Model file for the job. Use its own axes, mm. Face numbers are marked on the shaded views. A direction names the side the tool comes from. Round coordinates to 2 decimals unless told otherwise and drop trailing zeros. Write each loop counter-clockwise with the first axis right and the second up, starting at its lowest first coordinate (ties: lowest second). Pieces come first, ordered by that corner, then holes.
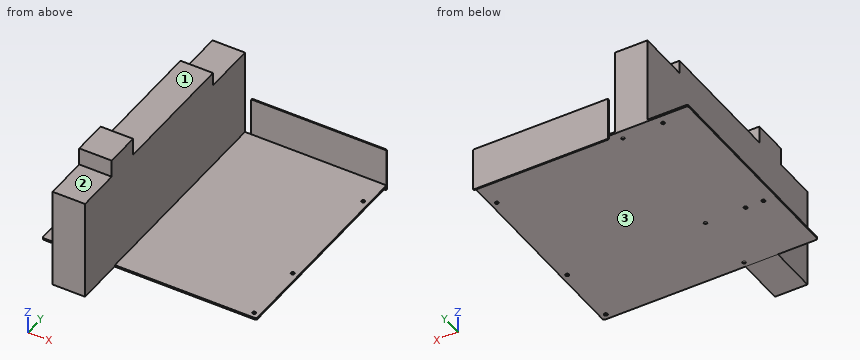
Autodesk Inventor part; units mm, degrees
ref_plane "YZ Plane" through (0, 0, 0) normal (1, 0, 0) x (0, 1, 0)
ref_plane "XZ Plane" through (0, 0, 0) normal (0, 1, 0) x (-1, 0, 0)
ref_plane "XY Plane" through (0, 0, 0) normal (0, 0, 1) x (1, 0, 0)
sketch "Sketch1" plane through (0, 0, 0) normal (0, 0, 1) x (1, 0, 0)
  line L0 (-122, 122) -> (122, 122)
  line L1 (122, 122) -> (122, -122)
  line L2 (122, -122) -> (-122, -122)
  line L3 (-122, -122) -> (-122, 122)
  point P0 (0, 0)
  dimension "d0" = 244
  dimension "d1" = 244
  dimension "d2" = 122
  dimension "d3" = 122
extrude "Extrusion1" add sketch "Sketch1" along normal blind 2
sketch "Sketch3" plane through (0, 0, 2) normal (0, 0, 1) x (1, 0, 0)
  line L0 (122, 122) -> (-122, 122)
  line L1 (-122, 122) -> (-122, -122)
  line L2 (-122, -122) -> (122, -122)
  line L3 (122, -122) -> (122, 122)
  line L4 (-209.7818, 111.84) -> (205.7988, 111.84) construction
  line L5 (-179.0523, -43.1) -> (193.3606, -43.1) construction
  line L6 (-192.2221, -115.49) -> (227.0168, -115.49) construction
  line L7 (115.49, -184.6971) -> (115.49, 232.3468) construction
  line L8 (-41.99, -199.0105) -> (-41.99, 288.2767) construction
  point P0 (0, 0)
  point P1 (-87.71, 111.84)
  point P2 (-41.99, 111.84)
  point P3 (-108.03, -43.1)
  point P4 (-87.71, -43.1)
  point P5 (-41.99, -43.1)
  point P6 (115.49, -43.1)
  point P7 (115.49, -115.49)
  point P8 (-41.99, -115.49)
  point P9 (115.49, 88.98)
  dimension "d12" = 34.29
  dimension "d13" = 20.32
  dimension "d18" = 10.16
  dimension "d20" = 227.33
  dimension "d22" = 90
  dimension "d23" = 22.86
  dimension "d24" = 154.94
  dimension "d25" = 45.72
  dimension "d26" = 203.2
  dimension "d27" = 45.72
hole "Hole1" at (-87.71, 111.84, 2) at (-41.99, 111.84, 2) at (-108.03, -43.1, 2) at (-87.71, -43.1, 2) at (-41.99, -43.1, 2) at (115.49, -43.1, 2) at (115.49, -115.49, 2) at (-41.99, -115.49, 2) at (115.49, 88.98, 2) direction (0, 0, -1) diameter 3.96 end through all
fillet "Fillet1" radius 2 4 edges at (-122, 122, 1) (-122, -122, 1) (122, -122, 1) (122, 122, 1)
sketch "Sketch4" plane through (-120, 122, 0) normal (0, 1, 0) x (1, 0, 0)
  line L0 (34.27, -2) -> (30.31, -2) construction
  line L1 (32.29, -21.9524) -> (32.29, 25.1381) construction
  line L2 (241.79, -45.39) -> (87.79, -45.39)
  line L3 (87.79, -45.39) -> (87.79, 4.35)
  line L4 (87.79, 4.35) -> (241.79, 4.35)
  line L5 (241.79, 4.35) -> (241.79, -45.39)
  line L6 (240, -2) -> (0, -2) construction
  line L7 (34.27, -2) -> (30.31, -2) construction
  point P0 (120, 0)
  point P1 (32.29, -2)
  dimension "d36" = 154
  dimension "d37" = 49.74
  dimension "d38" = 55.5
  dimension "d39" = 6.35
extrude "Extrusion3" add sketch "Sketch4" along normal blind 1.32
fillet "Fillet2" radius 1 4 edges at (121.79, 122.66, 45.39) (-32.21, 122.66, 45.39) (121.79, 122.66, -4.35) (-32.21, 122.66, -4.35)
sketch "Sketch5" plane through (-120, 122, 2) normal (0, 1, 0) x (1, 0, 0)
  line L0 (80.79, -98.65) -> (43.79, -98.65)
  line L1 (43.79, -98.65) -> (43.79, 1.35)
  line L2 (43.79, 1.35) -> (80.79, 1.35)
  line L3 (80.79, 1.35) -> (80.79, -98.65)
  line L4 (87.79, 5.35) -> (87.79, -42.39)
  line L5 (240.79, 6.35) -> (88.79, 6.35)
  point P0 (120, 2)
  dimension "d43" = 37
  dimension "d44" = 100
  dimension "d45" = 7
  dimension "d46" = 5
extrude "Extrusion4" add sketch "Sketch5" against normal blind 300
sketch "Sketch7" plane through (-120, -178, 2) normal (0, -1, 0) x (1, 0, 0)
  line L0 (43.79, 114) -> (80.79, 114)
  line L1 (80.79, 114) -> (80.79, 0)
  line L2 (80.79, 0) -> (43.79, 0)
  line L3 (43.79, 0) -> (43.79, 114)
  point P0 (120, -2)
  dimension "d49" = 37
  dimension "d50" = 114
extrude "Extrusion5" add sketch "Sketch7" against normal blind 240
sketch "Sketch8" plane through (-76.21, -178, 116) normal (0, 0, 1) x (1, 0, 0)
  line L0 (37, 0) -> (37, 240)
  line L1 (0, 0) -> (0, 240)
  line L2 (37, 90) -> (0, 90)
  line L3 (0, 90) -> (0, 50)
  line L4 (0, 50) -> (37, 50)
  line L5 (37, 50) -> (37, 90)
  line L6 (0, 0) -> (37, 0)
  point P0 (76.21, 178)
  dimension "d53" = 50
  dimension "d54" = 40
extrude "Extrusion6" add sketch "Sketch8" along normal blind 20 contours L4 L1 L2 L0
properties part number "Mobo"
1) Cut at B-B on y = 58. List the corners of the cut face in (x, z), and give its area (3 significant figures).
2) Cut at A-A on z = 30.5. List the corners of the cut face in (x, y).
3) Cut at D-D on z = 49. List the corners of the cut face in (x, y).
4) Wall check: probe 1 along X at (y, z) = (-43, 1); probe 2 along Y at (x, z) = (-87.71, 0.5); probe 3 along X at (y, z) = (111.84, 0.3). Give the ranges that are in metal, low to high.
5) Flat gauge pins, fed straight in: pin 1 Ø0.7 at (y, z) = (123, 31) entering from +X; pin 2 Ø2 at (x, y) = (-41.5, -44) entering from -Z; pin 3 Ø23 at (x, y) = (-108, 10) entering from +Z. Where does each tip first touch, or does it go through?
6) Cut at C-C on x = -19. List the corners of the cut face in (y, z).
7) Which spindle directions (+Z, -Z, +X, -X, +Y, -Y) get a long thin tool onto all of the face, cutting with end or side? Do the marked faces 1, 2 and 3. Say none if no direction does.
Result sheet:
1. outline: (-122, 0) - (122, 0) - (122, 2) - (-39.21, 2) - (-39.21, 116) - (-76.21, 116) - (-76.21, 2) - (-122, 2) - close
1. area: 4,710 mm2
2. outline: (-76.21, -178) - (-39.21, -178) - (-39.21, 122) - (-76.21, 122) - close; (-32.21, 122) - (121.79, 122) - (121.79, 123.32) - (-32.21, 123.32) - close
3. outline: (-76.21, -178) - (-39.21, -178) - (-39.21, 122) - (-76.21, 122) - close
4. probe 1: x = -122 to -110.01, -106.05 to -89.69, -85.73 to 113.51, 117.47 to 122
4. probe 2: y = -122 to -45.08, -41.12 to 109.86, 113.82 to 122
4. probe 3: x = -122 to -89.69, -85.73 to -43.97, -40.01 to 122
5. pin 1: stops at x = 121.79
5. pin 2: stops at z = 0
5. pin 3: stops at z = 2
6. outline: (-122, 0) - (122, 0) - (122, -4.35) - (123.32, -4.35) - (123.32, 45.39) - (122, 45.39) - (122, 2) - (-122, 2) - close
7. face 1: +Z, +X, -X, +Y
7. face 2: +Z, +X, -X, -Y
7. face 3: -Z, +X, -X, -Y
